Verification items for this drawing (mm, ordinates from the low corner). A direction names the side the tool comes from. Round coordinates to 2 decimals unless told otherwise and drop trailing zeros. Write each loop counter-clockwise with the first axis right and the second up, starting at its lowest first coordinate (ties: lowest second). Pieces come first, ordered by that corner, then holes.
Item 1: Cross-section at D-D (y = 4). Enter the section's corners in (x, z) (3 decimals), then the cut area to 3 significant figures.
Item 2: Depth check by flat-ended pin: P1, Ø7.5, axis at x = 21, z = 34, coming from the +Y side. Enter the tip coordinate at first touch or a pass-through.
Item 3: Access from +Z, -Z, +X, -X, +Y, -Y to the whole of each face (thin tool, end or side, straight path). Record for the marked faces 1 and 2.
Item 4: Cross-section at A-A (x = 20). Enter the section's corners in (y, z).
Item 5: Draft check along X on the marked faces 3, 4, 5 and 6. Enter one of: pulls with the +X half, pulls with the -X half, needs draft (parallel to the pull), parting line crosses it, or undercut.
Item 6: Cross-section at C-C (y = 1). Enter the section's corners in (x, z) (3 decimals).
Item 7: Scan lines: probe 1 along Z at (x, y) = (18.5, 10); probe 2 along X at (y, z) = (9.5, 43.5); probe 3 along Y at (x, z) = (32.5, 34). Record each from-to range of solid material in increasing order.
Item 8: Cross-section at B-B (z = 20). Enter the section's corners in (x, y), then the cut area to 3 significant figures.
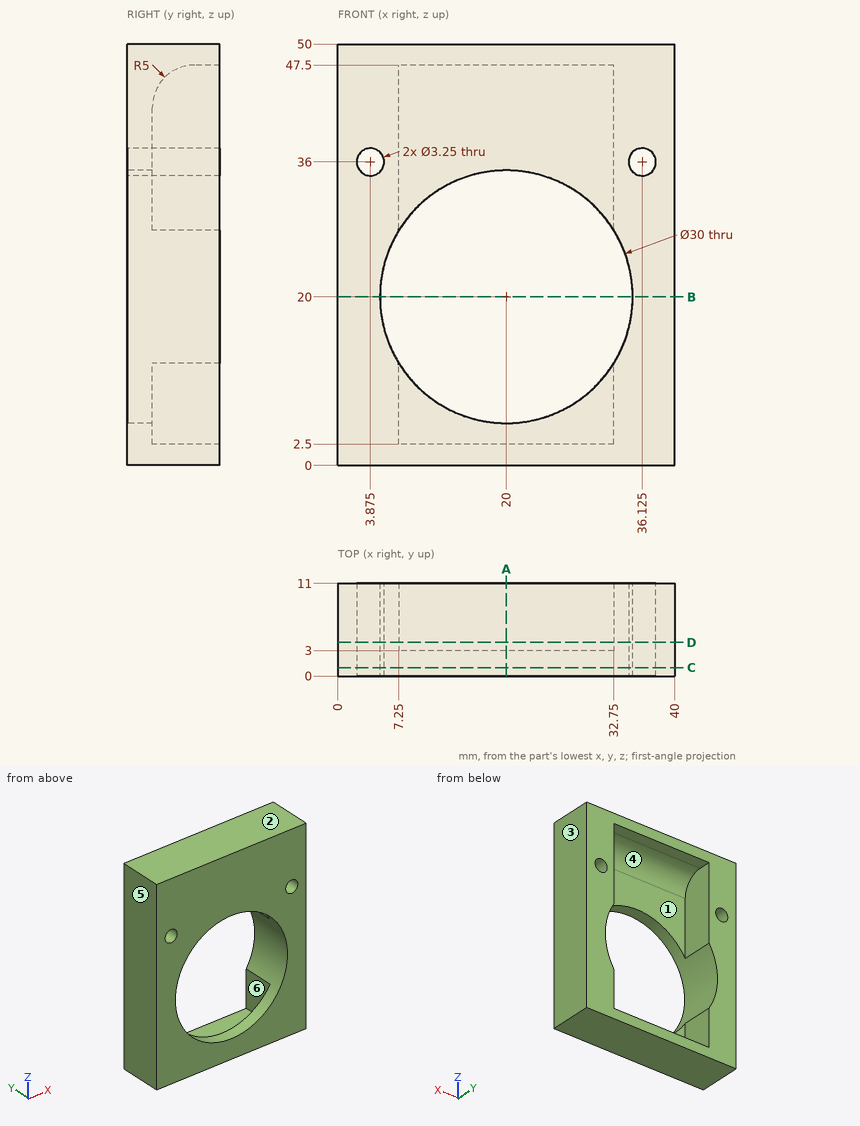
Resolved:
1. outline: (0, 0) - (40, 0) - (40, 50) - (0, 50) - close; hole circle Ø3.25 at (3.875, 36); hole (7.25, 2.5) - (32.75, 2.5) - (32.75, 12.098) arc R15 ccw to (32.75, 27.902) - (32.75, 45.5) - (7.25, 45.5) - (7.25, 27.902) arc R15 ccw to (7.25, 12.098) - close; hole circle Ø3.25 at (36.125, 36)
1. area: 839 mm2
2. P1: stops at y = 3
3. face 1: +Y
3. face 2: +Z, +X, -X, +Y, -Y
4. outline: (0, 0) - (11, 0) - (11, 2.5) - (3, 2.5) - (3, 5) - (0, 5) - close; (0, 35) - (3, 35) - (3, 42.5) arc R5 cw to (8, 47.5) - (11, 47.5) - (11, 50) - (0, 50) - close
5. face 3: pulls with the +X half
5. face 4: undercut
5. face 5: pulls with the -X half
5. face 6: undercut
6. outline: (0, 0) - (40, 0) - (40, 50) - (0, 50) - close; hole circle Ø3.25 at (3.875, 36); hole circle Ø30 at (20, 20); hole circle Ø3.25 at (36.125, 36)
7. probe 1: z = 0 to 2.5, 47.5 to 50
7. probe 2: x = 0 to 7.25, 32.75 to 40
7. probe 3: y = 0 to 3
8. outline: (0, 0) - (5, 0) - (5, 11) - (0, 11) - close; (35, 0) - (40, 0) - (40, 11) - (35, 11) - close
8. area: 110 mm2
